Build history of the part. All positions in model axes, mm. A direction names the side the tool comes from. Give positions to 0.01 mm unless a question says otherwise; leave off trailing zeros. Loops run counter-clockwise (first coordinate to the right, second up) from the corner with the lowest first, then second, coordinate; pieces in that order, holes last. Notation, with made-up numbers: (35, -23.75) -> (86, -23.75) arc R19 ccw to (86, 13.25) -> close; hole circle Ø7 at (71.5, 63.5). An arc over 180 degrees is marked (long way). Answer as a JSON object with one key per item and string values. Group by question number.
Q1. Band-saw the part on D-D, the plane z = -5. Write the cut outline in (x, y).
Q2. Two-plate mould, pull along Z, no slides. Class faces 1 (the cylindrical face through (-32.44, 1.97, -6.06)), 2 (the conical face through (-22.377, 2.759, -20.371)), 3 (the flat face through (4, 4, -23)), 4 (the flat face through (20, 2, 33)): pulls with the +Z half, pulls with the -Z half, needs draft (parallel to the pull), parting line crosses it, or undercut.
Q3. Band-saw the part on B-B, the plane z = 28. Write the cut outline in (x, y) (3 decimals), plus the area to 3 significant figures.
Q4. Band-saw the part on C-C, the plane x = -28. Write the cut outline in (y, z) (3 decimals), plus the area to 3 significant figures.
Q5. Wall check: probe 1 along Z at (x, y) = (0.5, 3.25); probe 2 along X at (y, z) = (3.15, 28) (3 decimals); probe 3 along X at (y, z) = (1, 11). Give the ranges that are in metal, low to high. Write a range as from..to.
Q6. Tool access for faces 5 (the conical face through (-46.251, 2.759, -24.983)), 6 (the cylindrical face through (32.44, 1.97, 6.06)), 7 (the cylindrical face through (-33.14, 2.03, 41.29)), 8 (the cylindrical face through (-41.34, 2.03, -22.85)), 9 (the cylindrical face through (-19.594, 2.028, 31.608)): list every direction of +Z, -Z, +X, -X, +Y, -Y with a clear straight run to the whole face (end or side of a thin tool).
Q7. Drop flat-ended pins along their axis: pin 1 (10 mm diameter, centred on x = 45, z = 28, fed in from -Y) (3 decimals); pin 2 (4 mm diameter, centred on x = -45, z = -28, fed in from -Y); pin 3 (1.8 mm diameter, centred on x = 38.5, y = 1, fed in from -Z); pin 4 (6 mm diameter, centred on x = 19.8, z = 19.8, fed in from -Y). Give the stop position or say it passes through.
Q8. Band-saw the part on A-A, the plane x = 28. Write the cut outline in (y, z) (3 decimals).
from build123d import *

# Parameters (mm, degrees)
SKETCH1_R           = 23
SKETCH1_R_2         = 2.5
SKETCH1_R_3         = 3.125
BOSS_EXTRUDE1_DEPTH = 4
FILLET1_R           = 8
CHAMFER1_SIZE       = 2.9


with BuildPart() as part:
    # Sketch1 → Boss-Extrude1 (new body)
    with BuildSketch(Plane(origin=(0, 0, 0), x_dir=(1, 0, 0), z_dir=(0, 1, 0))):
        with BuildLine():
            Line((-41.68337521, 33), (0, 33))
            ThreePointArc((0, 33), (12.411234198, 30.577136322), (23, 23.664319132))
            Line((23, 23.664319132), (23, 41.68337521))
            ThreePointArc((23, 41.68337521), (28, 51), (33, 41.68337521))
            Line((33, 41.68337521), (33, 0))
            ThreePointArc((33, 0), (30.577136322, -12.411234198), (23.664319132, -23))
            Line((23.664319132, -23), (41.68337521, -23))
            ThreePointArc((41.68337521, -23), (51, -28), (41.68337521, -33))
            Line((41.68337521, -33), (0, -33))
            ThreePointArc((0, -33), (-12.411234198, -30.577136322), (-23, -23.664319132))
            Line((-23, -23.664319132), (-23, -41.68337521))
            ThreePointArc((-23, -41.68337521), (-28, -51), (-33, -41.68337521))
            Line((-33, -41.68337521), (-33, 0))
            ThreePointArc((-33, 0), (-30.577136322, 12.411234198), (-23.664319132, 23))
            Line((-23.664319132, 23), (-41.68337521, 23))
            ThreePointArc((-41.68337521, 23), (-51, 28), (-41.68337521, 33))
        make_face()
        with Locations(Location((0, 0, 0), (0, 0, 270))):
            Circle(SKETCH1_R, mode=Mode.SUBTRACT)
        with Locations(Location((-19.798989873, 19.798989873, 0), (0, 0, 270))):
            Circle(SKETCH1_R_2, mode=Mode.SUBTRACT)
        with Locations(Location((19.798989873, 19.798989873, 0), (0, 0, 270))):
            Circle(SKETCH1_R_2, mode=Mode.SUBTRACT)
        with Locations(Location((19.798989873, -19.798989873, 0), (0, 0, 270))):
            Circle(SKETCH1_R_2, mode=Mode.SUBTRACT)
        with Locations(Location((-19.798989873, -19.798989873, 0), (0, 0, 270))):
            Circle(SKETCH1_R_2, mode=Mode.SUBTRACT)
        with Locations(Location((-45, 28, 0), (0, 0, 270))):
            Circle(SKETCH1_R_3, mode=Mode.SUBTRACT)
        with Locations(Location((28, 45, 0), (0, 0, 270))):
            Circle(SKETCH1_R_3, mode=Mode.SUBTRACT)
        with Locations(Location((45, -28, 0), (0, 0, 270))):
            Circle(SKETCH1_R_3, mode=Mode.SUBTRACT)
        with Locations(Location((-28, -45, 0), (0, 0, 270))):
            Circle(SKETCH1_R_3, mode=Mode.SUBTRACT)
    extrude(amount=BOSS_EXTRUDE1_DEPTH)

    # Fillet1
    fillet1_edges = [part.edges().sort_by_distance(p)[0] for p in [
        (-41.68337521, 2, -33),
        (23, 2, -23.664319132),
        (23, 2, -41.68337521),
        (33, 2, -41.68337521),
        (23.664319132, 2, 23),
        (41.68337521, 2, 23),
        (41.68337521, 2, 33),
        (-23, 2, 23.664319132),
        (-23, 2, 41.68337521),
        (-33, 2, 41.68337521),
        (-23.664319132, 2, -23),
        (-41.68337521, 2, -23),
    ]]
    fillet(fillet1_edges, radius=FILLET1_R)

    # Chamfer1
    # the kernel refuses this chamfer: 2.9 mm, written as the material it takes off along each edge
    with BuildSketch(Plane(origin=(-45, 0, -28), x_dir=(0, 0, 1), z_dir=(-1, 0, 0))) as chamfer1_piece_1:
        Polygon((3.125 + CHAMFER1_SIZE, 0), (3.125, CHAMFER1_SIZE), (3.125, 0), align=None)
    revolve(axis=Axis((-45, 0, -28), (0, 1, 0)), mode=Mode.SUBTRACT)
    with BuildSketch(Plane(origin=(-28, 0, 45), x_dir=(0, 0, 1), z_dir=(-1, 0, 0))) as chamfer1_piece_2:
        Polygon((3.125 + CHAMFER1_SIZE, 0), (3.125, CHAMFER1_SIZE), (3.125, 0), align=None)
    revolve(axis=Axis((-28, 0, 45), (0, 1, 0)), mode=Mode.SUBTRACT)
    with BuildSketch(Plane(origin=(45, 0, 28), x_dir=(0, 0, 1), z_dir=(-1, 0, 0))) as chamfer1_piece_3:
        Polygon((3.125 + CHAMFER1_SIZE, 0), (3.125, CHAMFER1_SIZE), (3.125, 0), align=None)
    revolve(axis=Axis((45, 0, 28), (0, 1, 0)), mode=Mode.SUBTRACT)
    with BuildSketch(Plane(origin=(28, 0, -45), x_dir=(0, 0, 1), z_dir=(-1, 0, 0))) as chamfer1_piece_4:
        Polygon((3.125 + CHAMFER1_SIZE, 0), (3.125, CHAMFER1_SIZE), (3.125, 0), align=None)
    revolve(axis=Axis((28, 0, -45), (0, 1, 0)), mode=Mode.SUBTRACT)
    with BuildSketch(Plane(origin=(19.798989873, 0, -19.798989873), x_dir=(0, 0, 1), z_dir=(-1, 0, 0))) as chamfer1_piece_5:
        Polygon((2.5 + CHAMFER1_SIZE, 0), (2.5, CHAMFER1_SIZE), (2.5, 0), align=None)
    revolve(axis=Axis((19.798989873, 0, -19.798989873), (0, 1, 0)), mode=Mode.SUBTRACT)
    with BuildSketch(Plane(origin=(19.798989873, 0, 19.798989873), x_dir=(0, 0, 1), z_dir=(-1, 0, 0))) as chamfer1_piece_6:
        Polygon((2.5 + CHAMFER1_SIZE, 0), (2.5, CHAMFER1_SIZE), (2.5, 0), align=None)
    revolve(axis=Axis((19.798989873, 0, 19.798989873), (0, 1, 0)), mode=Mode.SUBTRACT)
    with BuildSketch(Plane(origin=(-19.798989873, 0, 19.798989873), x_dir=(0, 0, 1), z_dir=(-1, 0, 0))) as chamfer1_piece_7:
        Polygon((2.5 + CHAMFER1_SIZE, 0), (2.5, CHAMFER1_SIZE), (2.5, 0), align=None)
    revolve(axis=Axis((-19.798989873, 0, 19.798989873), (0, 1, 0)), mode=Mode.SUBTRACT)
    with BuildSketch(Plane(origin=(-19.798989873, 0, -19.798989873), x_dir=(0, 0, 1), z_dir=(-1, 0, 0))) as chamfer1_piece_8:
        Polygon((2.5 + CHAMFER1_SIZE, 0), (2.5, CHAMFER1_SIZE), (2.5, 0), align=None)
    revolve(axis=Axis((-19.798989873, 0, -19.798989873), (0, 1, 0)), mode=Mode.SUBTRACT)

    # Chamfer2
    # the kernel refuses this chamfer: 1 mm, written as the material it takes off along each edge
    with BuildSketch(Plane(origin=(15, 0, -39.803847577), x_dir=(1, 0, 0), z_dir=(0, 0, 1))) as chamfer2_piece_1:
        with BuildLine():
            Line((9.028284271, -0.028284271), (7.971715729, 1.028284271))
            Line((7.971715729, 1.028284271), (7.951715729, 1.028284271))
            ThreePointArc((7.951715729, 1.028284271), (7.98, 0.514142136), (7.98, 0))
            Line((7.98, 0), (8, -0.02))
            ThreePointArc((8, -0.02), (8.514142136, -0.02), (9.028284271, -0.048284271))
            Line((9.028284271, -0.048284271), (9.028284271, -0.028284271))
        make_face()
    revolve(axis=Axis((15, 0, -39.803847577), (0, 1, 0)), revolution_arc=63.022782151, mode=Mode.SUBTRACT)
    with BuildSketch(Plane(origin=(23, 0, -38.157568057), x_dir=(0.9996219169112968, -0.02749587661058639, 0), z_dir=(0, 0, -1))) as chamfer2_piece_2:
        with BuildLine():
            Line((1.028673195, 0), (-0.056547155, -1.027117794))
            Line((-0.056547155, -1.027117794), (-0.076539593, -1.026567876))
            ThreePointArc((-0.076539593, -1.026567876), (-0.034129227, -0.51339783), (-0.019992438, 0.000549918))
            Line((-0.019992438, 0.000549918), (0.000549918, 0.019992438))
            ThreePointArc((0.000549918, 0.019992438), (0.514497665, 0.00585565), (1.029223113, 0.019992438))
            Line((1.029223113, 0.019992438), (1.028673195, 0))
        make_face()
    extrude(amount=1.646279521, mode=Mode.SUBTRACT)
    with BuildSketch(Plane(origin=(15, 0, -38.157568057), x_dir=(-0.3658536585365853, 0, 0.9306723916262885), z_dir=(-0.9306723916262885, 0, -0.3658536585365853))) as chamfer2_piece_3:
        with BuildLine():
            Line((9.028284271, -0.028284271), (7.971715729, 1.028284271))
            Line((7.971715729, 1.028284271), (7.951715729, 1.028284271))
            ThreePointArc((7.951715729, 1.028284271), (7.98, 0.514142136), (7.98, 0))
            Line((7.98, 0), (8, -0.02))
            ThreePointArc((8, -0.02), (8.514142136, -0.02), (9.028284271, -0.048284271))
            Line((9.028284271, -0.048284271), (9.028284271, -0.028284271))
        make_face()
    revolve(axis=Axis((15, 0, -38.157568057), (0, 1, 0)), revolution_arc=111.460127749, mode=Mode.SUBTRACT)
    with BuildSketch(Plane(origin=(0, 0, 0), x_dir=(0, 0, -1), z_dir=(-1, 0, 0))) as chamfer2_piece_4:
        with BuildLine():
            Line((31.971715729, 0.028284271), (33.028284271, -1.028284271))
            Line((33.028284271, -1.028284271), (33.048284271, -1.028284271))
            ThreePointArc((33.048284271, -1.028284271), (33.02, -0.514142136), (33.02, 0))
            Line((33.02, 0), (33, 0.02))
            ThreePointArc((33, 0.02), (32.485857864, 0.02), (31.971715729, 0.048284271))
            Line((31.971715729, 0.048284271), (31.971715729, 0.028284271))
        make_face()
    revolve(axis=Axis((0, 0, 0), (0, -1, 0)), revolution_arc=21.460127749, mode=Mode.SUBTRACT)
    with BuildSketch(Plane(origin=(-39.803847577, 0, -41), x_dir=(0, 0, 1), z_dir=(1, 0, 0))) as chamfer2_piece_5:
        with BuildLine():
            Line((9.028284271, 0.028284271), (7.971715729, -1.028284271))
            Line((7.971715729, -1.028284271), (7.951715729, -1.028284271))
            ThreePointArc((7.951715729, -1.028284271), (7.98, -0.514142136), (7.98, 0))
            Line((7.98, 0), (8, 0.02))
            ThreePointArc((8, 0.02), (8.514142136, 0.02), (9.028284271, 0.048284271))
            Line((9.028284271, 0.048284271), (9.028284271, 0.028284271))
        make_face()
    revolve(axis=Axis((-39.803847577, 0, -41), (0, -1, 0)), revolution_arc=63.022782151, mode=Mode.SUBTRACT)
    with BuildSketch(Plane(origin=(-39.803847577, 0, -33), x_dir=(0, 0.9996219169112968, -0.02749587661058908), z_dir=(1, 0, 0))) as chamfer2_piece_6:
        with BuildLine():
            Line((1.028673195, 0), (-0.056547155, 1.027117794))
            Line((-0.056547155, 1.027117794), (-0.076539593, 1.026567876))
            ThreePointArc((-0.076539593, 1.026567876), (-0.034129227, 0.51339783), (-0.019992438, -0.000549918))
            Line((-0.019992438, -0.000549918), (0.000549918, -0.019992438))
            ThreePointArc((0.000549918, -0.019992438), (0.514497665, -0.00585565), (1.029223113, -0.019992438))
            Line((1.029223113, -0.019992438), (1.028673195, 0))
        make_face()
    extrude(amount=39.803847577, mode=Mode.SUBTRACT)


solid = part.part
Worked answers:
{
 "1": {"outline": "(-32.62, 0) -> (-22.45, 0) -> (-22.45, 4) -> (-32.62, 4) -> close; (22.45, 0) -> (33, 0) -> (33, 4) -> (22.45, 4) -> close"},
 "2": {"face 1": "undercut", "face 2": "undercut", "face 3": "needs draft", "face 4": "pulls with the +Z half"},
 "3": {"outline": "(-33, 0) -> (38.975, 0) -> (41.875, 2.9) -> (41.875, 4) -> (-33, 4) -> close; (48.125, 2.9) -> (51, 0.025) -> (51, 4) -> (48.125, 4) -> close", "area": "303 mm2"},
 "4": {"outline": "(0, -32) -> (1, -33) -> (4, -33) -> (4, 41.875) -> (2.9, 41.875) -> (0, 38.975) -> close; (0.025, 51) -> (2.9, 48.125) -> (4, 48.125) -> (4, 51) -> close", "area": "302 mm2"},
 "5": {"probe 1": "-33..-22.99, 22.99..33", "probe 2": "-33..41.875, 48.125..51", "probe 3": "-33..-20.2, 20.2..31.11"},
 "6": {"face 5": "-Y", "face 6": "+X, +Y, -Y", "face 7": "-X, +Y, -Y", "face 8": "+Z, +Y, -Y", "face 9": "+Y, -Y"},
 "7": {"pin 1": "y = 1.025", "pin 2": "through", "pin 3": "z = 22.98", "pin 4": "y = 2.4"},
 "8": {"outline": "(0, -38.975) -> (2.9, -41.875) -> (4, -41.875) -> (4, 33) -> (0, 33) -> close; (0.025, -51) -> (4, -51) -> (4, -48.125) -> (2.9, -48.125) -> close"}
}
